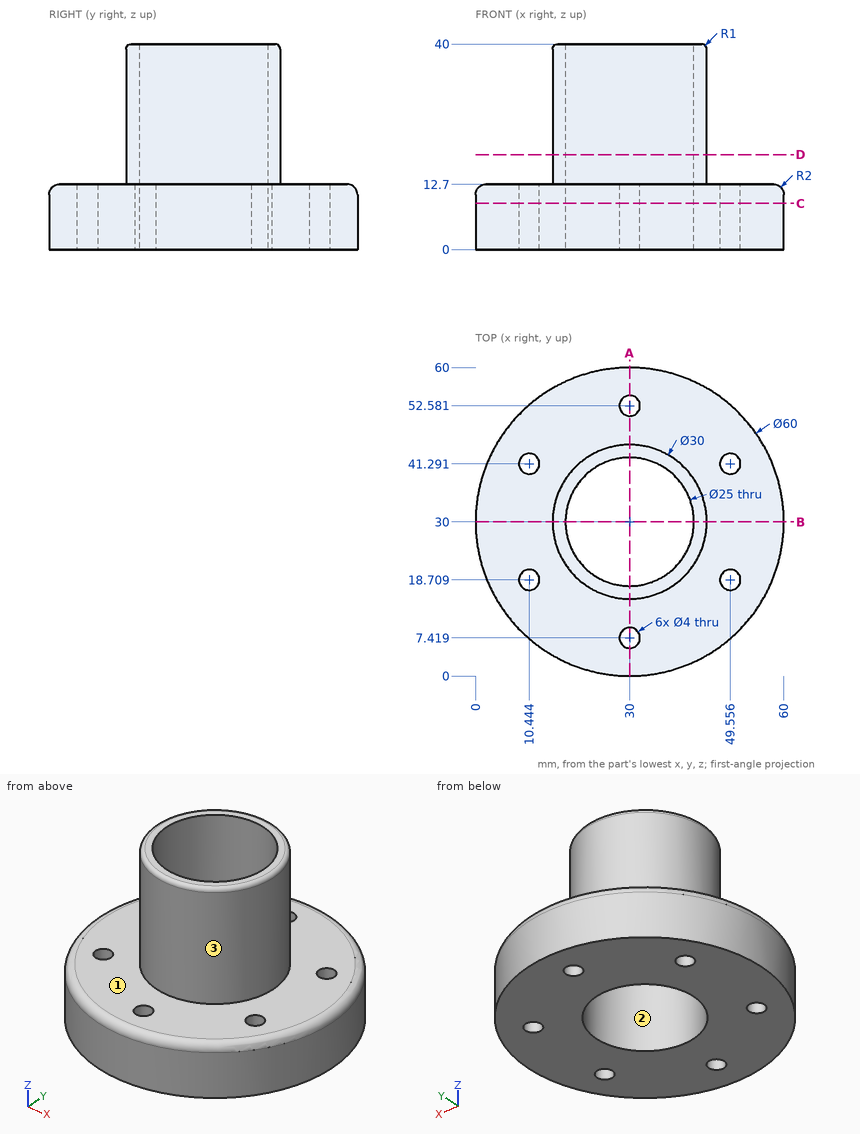
Design review of the part shown in the three views and the two pictorial views. Dimensions are in mm from the part's minimum x, y and z. Give positions to 0.01 mm unless a question says otherwise; leave off trailing zeros. Loops run counter-clockwise (first coordinate to the right, second up) from the corner with the lowest first, then second, coordinate; pieces in that order, holes last. Notation, with made-up numbers: (23.25, 10) - (79.25, 10) arc R24 cw to (79.25, 24) - close; hole circle Ø4 at (35, -22.5). An arc over 180 degrees is marked (long way). Use CSV: the item, a comma, the result in double quotes. Start each with the question number.
1. Draft analysis for pull direction X (two halves, no side actions). For the marked faces 1, 2 and 3, state which applies: released by +X, released by -X, zero draft, split by the parting line, or undercut.
2. Add section A-A (x = 30). State the section outline as (y, z) points.
3. Wall thickness on L1, parallel to Y at x = 30, z = 3.5; L2, parallel to Z at x = 18, y = 4.5; L3, parallel to Y at x = 19, z = 32.5 (1 decimal): over which ranges is each line inside the solid? List them lowest first.
4. Add section D-D (z = 18.5). State the section outline as (x, y) points, plus the area to 3 significant figures.
5. Add section C-C (z = 9). State the section outline as (x, y) points (1 decimal), plus the area to 3 significant figures.
6. Add section B-B (y = 30). State the section outline as (x, z) points, plus the area to 3 significant figures.
7. Insertion check: P1, Ø6, axis at y = 42.5, z = 28, coming from the -X side; P2, Ø1, axis at y = 17.5, z = 15.5, coming from the +X side; P3, Ø6, axis at y = 20.5, z = 15, coming from the +X side (1 decimal); P4, Ø4, axis at x = 25, y = 10.5, coming from the -Z side. Each pin has a flat end and moves straight along its axis. Give the tip position at first contact, or say it passes through.
Results found:
1,face 1,"zero draft"
1,face 2,"undercut"
1,face 3,"split by the parting line"
2,outline,"(0, 0) - (5.42, 0) - (5.42, 12.7) - (2, 12.7) arc R2 ccw to (0, 10.7) - close; (9.42, 0) - (17.5, 0) - (17.5, 40) - (16, 40) arc R1 ccw to (15, 39) - (15, 12.7) - (9.42, 12.7) - close; (42.5, 0) - (50.58, 0) - (50.58, 12.7) - (45, 12.7) - (45, 39) arc R1 ccw to (44, 40) - (42.5, 40) - close; (54.58, 0) - (60, 0) - (60, 10.7) arc R2 ccw to (58, 12.7) - (54.58, 12.7) - close"
3,L1,"y = 0 to 5.42, 9.42 to 17.5, 42.5 to 50.58, 54.58 to 60"
3,L2,"z = 0 to 12.69"
3,L3,"y = 19.8 to 24.1, 35.9 to 40.2"
4,outline,"circle Ø30 at (30, 30); hole circle Ø25 at (30, 30)"
4,area,"216 mm²"
5,outline,"circle Ø60 at (30, 30); hole circle Ø4 at (10.4, 18.7); hole circle Ø4 at (10.4, 41.3); hole circle Ø25 at (30, 30); hole circle Ø4 at (30, 7.4); hole circle Ø4 at (30, 52.6); hole circle Ø4 at (49.6, 18.7); hole circle Ø4 at (49.6, 41.3)"
5,area,"2,260 mm²"
6,outline,"(0, 0) - (17.5, 0) - (17.5, 40) - (16, 40) arc R1 ccw to (15, 39) - (15, 12.7) - (2, 12.7) arc R2 ccw to (0, 10.7) - close; (42.5, 0) - (60, 0) - (60, 10.7) arc R2 ccw to (58, 12.7) - (45, 12.7) - (45, 39) arc R1 ccw to (44, 40) - (42.5, 40) - close"
6,area,"579 mm²"
7,P1,"stops at x = 18.39"
7,P2,"stops at x = 39"
7,P3,"stops at x = 58.1"
7,P4,"stops at z = 0"
